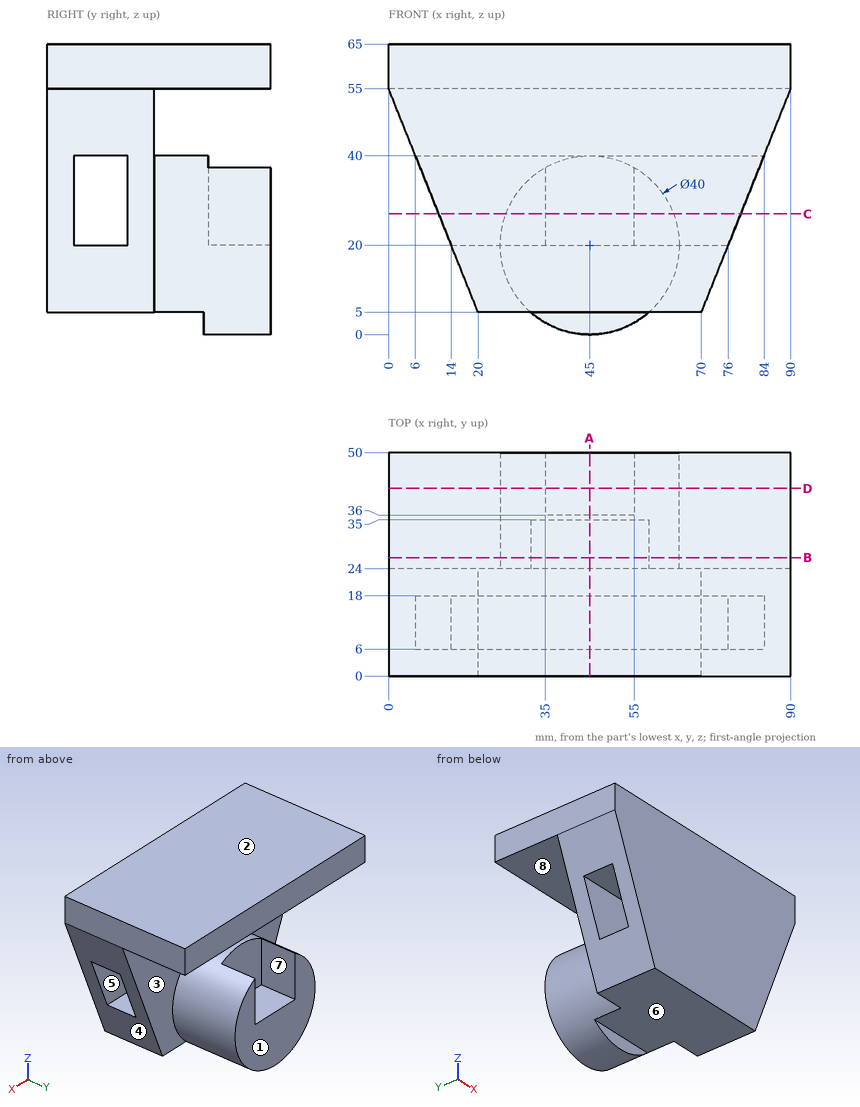
Check sheet for the drawn part. Datum: minimum x, y, z corner. Units: mm. A direction names the side the tool comes from. Coordinates: 2 decimals unless noted, no trailing zeros. Order: outer loops, then holes, each group sorted by start corner. A loop starts at its lowest first (then second) coordinate and runs counter-clockwise, first axis right, second up. Notation, with made-up numbers: (50, 72.5) -> (77, 72.5) arc R20 cw to (77, 88.5) -> close; hole circle Ø6 at (14, 57). An arc over 180 degrees is marked (long way). Use a Markdown table: item, result. Add a question column.
1. Cross-section at B-B (y = 26.5). Enter the section's corners in (x, z), and give its area (3 significant figures).
2. Mould release check, pull along Z, two halves, no side actions. Record for the marked faces 1, 2 and 3: pulls with the +Z half, pulls with the -Z half, needs draft (parallel to the pull), parting line crosses it, or undercut.
3. Cross-section at D-D (y = 42). Enter the section's corners in (x, z), and give its area (3 significant figures).
4. Go/stop test with flat-tipped pins: pin 1 Ø11 at (y, z) = (44, 24.5) entering from +X; pin 2 Ø11 at (y, z) = (40, 31.5) entering from -X; pin 3 Ø6 at (x, z) = (59.5, 30) entering from -Y; pin 4 Ø1 at (x, z) = (65.5, 15.5) entering from +Y. Record where each tip stops, or that it passes through.
5. Set-up check for the marked faces 4, 5, 6, 7 and 8: record each of +Z, -Z, +X, -X, +Y, -Y from which the full face is reachable in a straight line by a thin tool's end or side.
6. Cross-section at C-C (z = 27). Enter the section's corners in (x, y) (3 decimals), and give its area (3 significant figures).
7. Cross-section at A-A (x = 45). Enter the section's corners in (y, z), and give its area (4 significant figures).
8. Material ranges on L1, parallel to Y at x = 79, z = 30; L2, parallel to Z at x = 76, y = 34; L3, parallel to Z at x = 14, y = 3, recorded low to high.
Filled sheet:
| question | item | result |
|---|---|---|
| 1 | outline | (0, 55) -> (90, 55) -> (90, 65) -> (0, 65) -> close; (31.77, 5) -> (58.23, 5) arc R20 ccw (long way) to start |
| 1 | area | 2,070 mm2 |
| 2 | face 1 | needs draft |
| 2 | face 2 | pulls with the +Z half |
| 2 | face 3 | undercut |
| 3 | outline | (0, 55) -> (90, 55) -> (90, 65) -> (0, 65) -> close; (35, 20) -> (35, 37.32) arc R20 ccw (long way) to (55, 37.32) -> (55, 20) -> close |
| 3 | area | 1,770 mm2 |
| 4 | pin 1 | x = 65 |
| 4 | pin 2 | x = 25.92 |
| 4 | pin 3 | y = 0 |
| 4 | pin 4 | y = 24 |
| 5 | face 4 | -Z, +X, +Y, -Y |
| 5 | face 5 | +X, -X |
| 5 | face 6 | -Z, +X, -X, -Y |
| 5 | face 7 | +Y |
| 5 | face 8 | +X, -X, +Y |
| 6 | outline | (11.2, 0) -> (78.8, 0) -> (78.8, 6) -> (11.2, 6) -> close; (11.2, 18) -> (78.8, 18) -> (78.8, 24) -> (63.735, 24) -> (63.735, 50) -> (55, 50) -> (55, 36) -> (35, 36) -> (35, 50) -> (26.265, 50) -> (26.265, 24) -> (11.2, 24) -> close |
| 6 | area | 1,510 mm2 |
| 7 | outline | (0, 5) -> (35, 5) -> (35, 0) -> (50, 0) -> (50, 20) -> (36, 20) -> (36, 40) -> (24, 40) -> (24, 55) -> (50, 55) -> (50, 65) -> (0, 65) -> close; hole (6, 20) -> (18, 20) -> (18, 40) -> (6, 40) -> close |
| 7 | area | 2,165 mm2 |
| 8 | L1 | 0 to 6, 18 to 24 |
| 8 | L2 | 55 to 65 |
| 8 | L3 | 20 to 65 |
